Part model, mm, in its own coordinate system. Face numbers are marked on the shaded views. A direction names the side the tool comes from. Coordinates: 2 decimals unless noted, no trailing zeros. Loops run counter-clockwise (first coordinate to the right, second up) from the corner with the lowest first, then second, coordinate; pieces in that order, holes last. Notation, with made-up numbers: (-7.75, -15) -> (18.25, -15) arc R21 ccw to (18.25, 14) -> close; hole circle Ø5 at (-21, 86). An arc over 180 degrees is marked (long way). One line per question, with ' | ' between items. Start each with the question number.
1) Cut at A-A (y = 11). List the corners of the cut face in (x, z), plus the area to 3 significant figures.
2) 3-axis set-ups, long thin cutter, end or side, ignore diameter. For the marked faces 4 and 5: which of +Z, -Z, +X, -X, +Y, -Y reach the whole face in a straight line?
3) Two-plate mould, pull along X, no slides. Class the marked faces 1, 2 and 3: released by +X, released by -X, zero draft, split by the parting line, or undercut.
4) Probe L1, parallel to X at y = 19.5, z = 29.5; L2, parallel to X at y = 10.25, z = -36; L3, parallel to Z at x = 46.5, y = 8.75. List the from-to ranges inside material, lowest first. Write a range as from..to.
5) Cut at D-D (y = 21.75). List the corners of the cut face in (x, z).
6) Drop flat-ended pins along their axis: pin 1 (3 mm diameter, centred on x = -53.5, z = 36, fed in from +Y); pin 2 (3 mm diameter, centred on x = 28.5, z = 27.5, fed in from +Y); pin 3 (1.6 mm diameter, centred on y = 24.5, z = -42, fed in from -X). Give the stop position or say it passes through.
7) Cut at B-B (z = -2). List the corners of the cut face in (x, y), plus the area to 3 significant figures.
8) Cut at C-C (x = 50.5). List the corners of the cut face in (y, z).
from build123d import *

# Parameters (mm, degrees)
SKETCH1_W           = 120
SKETCH1_H           = 85
BOSS_EXTRUDE1_DEPTH = 30
SKETCH2_W           = 83
SKETCH2_H           = 81
CUT_EXTRUDE1_DEPTH  = 29
SKETCH3_W           = 31
SKETCH3_H           = 81
CUT_EXTRUDE2_DEPTH  = 29
SKETCH4_W           = 35
SKETCH4_H           = 85
CUT_EXTRUDE3_DEPTH  = 10
SKETCH5_W           = 9
SKETCH5_H           = 9
SKETCH5_R           = 1.25
BOSS_EXTRUDE2_DEPTH = 19
SKETCH6_R           = 1.75
SKETCH6_R_2         = 1
BOSS_EXTRUDE3_DEPTH = 5
SKETCH7_W           = 5
SKETCH7_H           = 8.298973679
SKETCH7_R           = 0.9
BOSS_EXTRUDE4_DEPTH = 3
SKETCH8_R           = 3
CUT_EXTRUDE4_DEPTH  = 2
FILLET1_R           = 1


with BuildPart() as part:
    # Sketch1 → Boss-Extrude1 (new body)
    with BuildSketch(Plane(origin=(0, 0, 0), x_dir=(1, 0, 0), z_dir=(0, 1, 0))):
        Rectangle(SKETCH1_W, SKETCH1_H)
    extrude(amount=BOSS_EXTRUDE1_DEPTH)

    # Sketch2 → Cut-Extrude1 (cut)
    with BuildSketch(Plane(origin=(0, 30, 0), x_dir=(1, 0, 0), z_dir=(0, 1, 0))):
        with Locations((16.5, 0)):
            Rectangle(SKETCH2_W, SKETCH2_H)
    extrude(amount=-CUT_EXTRUDE1_DEPTH, mode=Mode.SUBTRACT)

    # Sketch3 → Cut-Extrude2 (cut)
    with BuildSketch(Plane(origin=(0, 30, 0), x_dir=(1, 0, 0), z_dir=(0, 1, 0))):
        with Locations((-42.5, 0)):
            Rectangle(SKETCH3_W, SKETCH3_H)
    extrude(amount=-CUT_EXTRUDE2_DEPTH, mode=Mode.SUBTRACT)

    # Sketch4 → Cut-Extrude3 (cut)
    with BuildSketch(Plane(origin=(0, 30, 0), x_dir=(1, 0, 0), z_dir=(0, 1, 0))):
        with Locations((-42.5, 0)):
            Rectangle(SKETCH4_W, SKETCH4_H)
    extrude(amount=-CUT_EXTRUDE3_DEPTH, mode=Mode.SUBTRACT)

    # Sketch5 → Boss-Extrude2 (add)
    # profile 1 of 4: a face of its own
    with BuildSketch(Plane(origin=(0, 1, 0), x_dir=(1, 0, 0), z_dir=(0, 1, 0))):
        with Locations((-31.5, 36)):
            Rectangle(SKETCH5_W, SKETCH5_H)
        with Locations(Location((-31.5, 36, 0), (0, 0, 270))):
            Circle(SKETCH5_R, mode=Mode.SUBTRACT)
    # profile 2 of 4: a face of its own
    with BuildSketch(Plane(origin=(0, 1, 0), x_dir=(1, 0, 0), z_dir=(0, 1, 0))):
        with Locations((-53.5, 36)):
            Rectangle(SKETCH5_W, SKETCH5_H)
        with Locations(Location((-53.5, 36, 0), (0, 0, 270))):
            Circle(SKETCH5_R, mode=Mode.SUBTRACT)
    # profile 3 of 4: a face of its own
    with BuildSketch(Plane(origin=(0, 1, 0), x_dir=(1, 0, 0), z_dir=(0, 1, 0))):
        with Locations((-31.5, -36)):
            Rectangle(SKETCH5_W, SKETCH5_H)
        with Locations(Location((-31.5, -36, 0), (0, 0, 270))):
            Circle(SKETCH5_R, mode=Mode.SUBTRACT)
    # profile 4 of 4: a face of its own
    with BuildSketch(Plane(origin=(0, 1, 0), x_dir=(1, 0, 0), z_dir=(0, 1, 0))):
        with Locations((-53.5, -36)):
            Rectangle(SKETCH5_W, SKETCH5_H)
        with Locations(Location((-53.5, -36, 0), (0, 0, 270))):
            Circle(SKETCH5_R, mode=Mode.SUBTRACT)
    extrude(amount=BOSS_EXTRUDE2_DEPTH)

    # Sketch6 → Boss-Extrude3 (add)
    # profile 1 of 4: a face of its own
    with BuildSketch(Plane(origin=(0, 1, 0), x_dir=(1, 0, 0), z_dir=(0, 1, 0))):
        with Locations(Location((-53, 26.5, 0), (0, 0, 270))):
            Circle(SKETCH6_R)
        with Locations(Location((-53, 26.5, 0), (0, 0, 270))):
            Circle(SKETCH6_R_2, mode=Mode.SUBTRACT)
    # profile 2 of 4: a face of its own
    with BuildSketch(Plane(origin=(0, 1, 0), x_dir=(1, 0, 0), z_dir=(0, 1, 0))):
        with Locations(Location((-32.000361852, 26.376721252, 0), (0, 0, 270))):
            Circle(SKETCH6_R)
        with Locations(Location((-32.000361852, 26.376721252, 0), (0, 0, 270))):
            Circle(SKETCH6_R_2, mode=Mode.SUBTRACT)
    # profile 3 of 4: a face of its own
    with BuildSketch(Plane(origin=(0, 1, 0), x_dir=(1, 0, 0), z_dir=(0, 1, 0))):
        with Locations(Location((-32.000361852, -6.623278748, 0), (0, 0, 270))):
            Circle(SKETCH6_R)
        with Locations(Location((-32.000361852, -6.623278748, 0), (0, 0, 270))):
            Circle(SKETCH6_R_2, mode=Mode.SUBTRACT)
    # profile 4 of 4: a face of its own
    with BuildSketch(Plane(origin=(0, 1, 0), x_dir=(1, 0, 0), z_dir=(0, 1, 0))):
        with Locations(Location((-53, -6.5, 0), (0, 0, 270))):
            Circle(SKETCH6_R)
        with Locations(Location((-53, -6.5, 0), (0, 0, 270))):
            Circle(SKETCH6_R_2, mode=Mode.SUBTRACT)
    extrude(amount=BOSS_EXTRUDE3_DEPTH)

    # Sketch7 → Boss-Extrude4 (add)
    with BuildSketch(Plane.ZY.offset(27)):
        with Locations((20.5, 5.14948684)):
            Rectangle(SKETCH7_W, SKETCH7_H)
        with Locations((20.5, 6.798973679)):
            Circle(SKETCH7_R, mode=Mode.SUBTRACT)
    extrude(amount=BOSS_EXTRUDE4_DEPTH)

    # Sketch8 → Cut-Extrude4 (cut)
    with BuildSketch(Plane.ZY.offset(27)):
        with Locations((20.5, 16.298973679)):
            Circle(SKETCH8_R)
    extrude(amount=-CUT_EXTRUDE4_DEPTH, mode=Mode.SUBTRACT)

    # Fillet1
    fillet1_edges = [part.edges().sort_by_distance(p)[0] for p in [
        (17.5, 30, 42.5),
        (-60, 10, 42.5),
    ]]
    fillet(fillet1_edges, radius=FILLET1_R)


solid = part.part
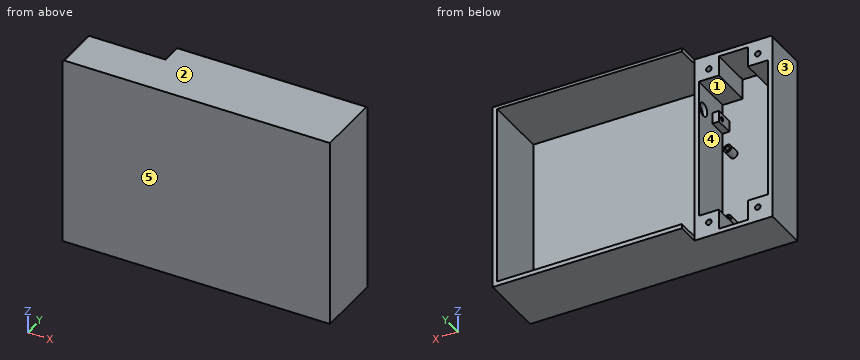
Reported:
1) outline: (-60, -42.5) -> (60, -42.5) -> (60, 42.5) -> (-59, 42.5) arc R1 ccw to (-60, 41.5) -> close; hole (-58, -31.5) -> (-49, -31.5) -> (-49, -40.5) -> (-36, -40.5) -> (-36, -31.5) -> (-27, -31.5) -> (-27, 31.5) -> (-36, 31.5) -> (-36, 40.5) -> (-49, 40.5) -> (-49, 31.5) -> (-58, 31.5) -> close; hole circle Ø2.5 at (-53.5, -36); hole circle Ø2.5 at (-53.5, 36); hole circle Ø2.5 at (-31.5, -36); hole circle Ø2.5 at (-31.5, 36); hole (-25, -40.5) -> (58, -40.5) -> (58, 40.5) -> (-25, 40.5) -> close | area: 1,270 mm²
2) face 4: +Y | face 5: +Z, -Z, +X, -X, -Y
3) face 1: undercut | face 2: zero draft | face 3: released by -X
4) L1: x = -60..-58, -27..-25, 58..60 | L2: x = -60..-54.75, -52.25..-49, -36..-32.75, -30.25..-25, 58..60 | L3: z = -42.5..-40.5, 40.5..42.5
5) outline: (-25, -42.5) -> (60, -42.5) -> (60, 42.5) -> (-25, 42.5) -> (-25, 40.5) -> (58, 40.5) -> (58, -40.5) -> (-25, -40.5) -> close
6) pin 1: stops at y = 20 | pin 2: stops at y = 1 | pin 3: stops at x = -25
7) outline: (-60, 0) -> (60, 0) -> (60, 30) -> (58, 30) -> (58, 1) -> (-25, 1) -> (-25, 20) -> (-27, 20) -> (-27, 1) -> (-58, 1) -> (-58, 20) -> (-60, 20) -> close | area: 254 mm²
8) outline: (0, -42.5) -> (30, -42.5) -> (30, -40.5) -> (1, -40.5) -> (1, 40.5) -> (30, 40.5) -> (30, 41.5) arc R1 ccw to (29, 42.5) -> (0, 42.5) -> close
